from build123d import *

# Parameters (mm, degrees)
EXTRUIR1_DEPTH            = 5.5
EXTRUIR2_DEPTH            = 2
EXTRUIR3_DEPTH            = 2
CROQUIS5_R                = 1
EXTRUIR4_DEPTH            = 41.608650556
VACIADO1_DEPTH            = 2
VACIADO1_START            = 2
VACIADO1_2_DEPTH          = 2
CROQUIS8_W                = 4
CROQUIS8_H                = 1
EXTRUIR7_DEPTH            = 3
SIMETR_A3_COPY_1_SKETCH_W = 4
SIMETR_A3_COPY_1_SKETCH_H = 1
SIMETR_A3_COPY_1_DEPTH    = 3
REDONDEO1_R               = 0.5
CROQUIS9_W                = 5
CROQUIS9_H                = 7.4
EXTRUIR8_DEPTH            = 41.707032562


# Read off the part's stored shape, not the designer's step: Vaciado1
with BuildPart() as part:
    # Croquis2 → Extruir1 (new body)
    with BuildSketch(Plane(origin=(0, 0, 0), x_dir=(0, 0, -1), z_dir=(1, 0, 0))):
        with BuildLine():
            Line((-37, 8.75), (37, 8.75))
            ThreePointArc((37, 8.75), (38.767766953, 8.017766953), (39.5, 6.25))
            Line((39.5, 6.25), (39.5, -6.25))
            ThreePointArc((39.5, -6.25), (38.767766953, -8.017766953), (37, -8.75))
            Line((37, -8.75), (-37, -8.75))
            ThreePointArc((-37, -8.75), (-38.767766953, -8.017766953), (-39.5, -6.25))
            Line((-39.5, -6.25), (-39.5, 6.25))
            ThreePointArc((-39.5, 6.25), (-38.767766953, 8.017766953), (-37, 8.75))
        make_face()
    extrude(amount=EXTRUIR1_DEPTH)

    # Croquis3 → Extruir2 (cut)
    with BuildSketch(Plane(origin=(5.5, 0, 0), x_dir=(0, 0, -1), z_dir=(1, 0, 0))):
        with BuildLine():
            Line((-32, 6.75), (32, 6.75))
            ThreePointArc((32, 6.75), (33.060660172, 6.310660172), (33.5, 5.25))
            Line((33.5, 5.25), (33.5, -5.25))
            ThreePointArc((33.5, -5.25), (33.060660172, -6.310660172), (32, -6.75))
            Line((32, -6.75), (-32, -6.75))
            ThreePointArc((-32, -6.75), (-33.060660172, -6.310660172), (-33.5, -5.25))
            Line((-33.5, -5.25), (-33.5, 5.25))
            ThreePointArc((-33.5, 5.25), (-33.060660172, 6.310660172), (-32, 6.75))
        make_face()
    extrude(amount=-EXTRUIR2_DEPTH, mode=Mode.SUBTRACT)

    # Croquis4 → Extruir3 (cut)
    with BuildSketch(Plane(origin=(5.5, 0, 0), x_dir=(0, 0, -1), z_dir=(1, 0, 0))):
        with BuildLine():
            Line((-39.5, 2.5), (-37.32, 2.5))
            ThreePointArc((-37.32, 2.5), (-34.82, 0), (-37.32, -2.5))
            Line((-37.32, -2.5), (-39.5, -2.5))
            Line((-39.5, -2.5), (-39.5, 2.5))
        make_face()
    extruir3 = extrude(amount=-EXTRUIR3_DEPTH, mode=Mode.SUBTRACT)

    # Croquis5 → Extruir4 (cut, through all)
    with BuildSketch(Plane(origin=(3.5, 0, 0), x_dir=(0, 0, -1), z_dir=(1, 0, 0))):
        with Locations((-37.32, 0)):
            Circle(CROQUIS5_R)
    extruir4 = extrude(amount=-EXTRUIR4_DEPTH, mode=Mode.SUBTRACT)

    # Simetría1: Extruir3, Extruir4 across plane
    add(extruir3.mirror(Plane.XY), mode=Mode.SUBTRACT)
    add(extruir4.mirror(Plane.XY), mode=Mode.SUBTRACT)

    # Vaciado1 outline → Vaciado1 (cut)
    with BuildSketch(Plane.YZ):
        with BuildLine():
            ThreePointArc((-7.25, -37), (-6.957106781, -37.707106781), (-6.25, -38))
            Line((-6.25, -38), (-2.405743128, -38))
            ThreePointArc((-2.405743128, -38), (0, -34.82), (2.405743128, -38))
            Line((2.405743128, -38), (6.25, -38))
            ThreePointArc((6.25, -38), (6.957106781, -37.707106781), (7.25, -37))
            Line((7.25, -37), (7.25, 37))
            ThreePointArc((7.25, 37), (6.957106781, 37.707106781), (6.25, 38))
            Line((6.25, 38), (2.405743128, 38))
            ThreePointArc((2.405743128, 38), (0, 34.82), (-2.405743128, 38))
            Line((-2.405743128, 38), (-6.25, 38))
            ThreePointArc((-6.25, 38), (-6.957106781, 37.707106781), (-7.25, 37))
            Line((-7.25, 37), (-7.25, -37))
        make_face()
    extrude(amount=VACIADO1_DEPTH, mode=Mode.SUBTRACT)

    # Vaciado1 2 outline → Vaciado1 2 (cut)
    with BuildSketch(Plane.YZ.offset(VACIADO1_START)):
        with BuildLine():
            Line((-7.25, -34.236067977), (-7.25, -37))
            ThreePointArc((-7.25, -37), (-6.957106781, -37.707106781), (-6.25, -38))
            Line((-6.25, -38), (-4, -38))
            Line((-4, -38), (-4, -37.32))
            ThreePointArc((-4, -37.32), (-3.810109158, -36.102187122), (-3.258465897, -35))
            Line((-3.258465897, -35), (-5.25, -35))
            ThreePointArc((-5.25, -35), (-6.320466269, -34.802517077), (-7.25, -34.236067977))
        make_face()
        with BuildLine():
            Line((-7.25, 37), (-7.25, 34.236067977))
            ThreePointArc((-7.25, 34.236067977), (-6.320466269, 34.802517077), (-5.25, 35))
            Line((-5.25, 35), (-3.258465897, 35))
            ThreePointArc((-3.258465897, 35), (-3.810109158, 36.102187122), (-4, 37.32))
            Line((-4, 37.32), (-4, 38))
            Line((-4, 38), (-6.25, 38))
            ThreePointArc((-6.25, 38), (-6.957106781, 37.707106781), (-7.25, 37))
        make_face()
        with BuildLine():
            Line((4, -37.32), (4, -38))
            Line((4, -38), (6.25, -38))
            ThreePointArc((6.25, -38), (6.957106781, -37.707106781), (7.25, -37))
            Line((7.25, -37), (7.25, -34.236067977))
            ThreePointArc((7.25, -34.236067977), (6.320466269, -34.802517077), (5.25, -35))
            Line((5.25, -35), (3.258465897, -35))
            ThreePointArc((3.258465897, -35), (3.810109158, -36.102187122), (4, -37.32))
        make_face()
        with BuildLine():
            Line((6.25, 38), (4, 38))
            Line((4, 38), (4, 37.32))
            ThreePointArc((4, 37.32), (3.810109158, 36.102187122), (3.258465897, 35))
            Line((3.258465897, 35), (5.25, 35))
            ThreePointArc((5.25, 35), (6.320466269, 34.802517077), (7.25, 34.236067977))
            Line((7.25, 34.236067977), (7.25, 37))
            ThreePointArc((7.25, 37), (6.957106781, 37.707106781), (6.25, 38))
        make_face()
    extrude(amount=VACIADO1_2_DEPTH, mode=Mode.SUBTRACT)

    # Croquis8 → Extruir7 (add)
    with BuildSketch(Plane.ZY.offset(-2)):
        with Locations((-20.5, 7.65)):
            Rectangle(CROQUIS8_W, CROQUIS8_H)
    extruir7 = extrude(amount=EXTRUIR7_DEPTH)

    # Simetría2: Extruir7 across plane
    add(extruir7.mirror(Plane.XY))

    # Simetría3: Extruir7 across plane
    add(extruir7.mirror(Plane.ZX))

    # Simetría3 copy 1 sketch → Simetría3 copy 1 (add)
    with BuildSketch(Plane(origin=(2, 0, 0), x_dir=(0, 0, -1), z_dir=(-1, 0, 0))):
        with Locations((-20.5, 7.65)):
            Rectangle(SIMETR_A3_COPY_1_SKETCH_W, SIMETR_A3_COPY_1_SKETCH_H)
    extrude(amount=SIMETR_A3_COPY_1_DEPTH)

    # Redondeo1
    redondeo1_edges = [part.edges().sort_by_distance(p)[0] for p in [
        (5.5, -8.017766953, 38.767766953),
        (5.5, -8.75, 0),
        (5.5, -8.017766953, -38.767766953),
        (5.5, -4.375, -39.5),
        (5.5, 8.017766953, -38.767766953),
        (5.5, 8.75, 0),
        (5.5, 8.017766953, 38.767766953),
        (5.5, -4.375, 39.5),
        (5.5, -2.5, 38.41),
        (5.5, 0, 34.82),
        (5.5, 2.5, 38.41),
        (5.5, 4.375, 39.5),
        (5.5, 4.375, -39.5),
        (5.5, -2.5, -38.41),
        (5.5, 0, -34.82),
        (5.5, 2.5, -38.41),
    ]]
    fillet(redondeo1_edges, radius=REDONDEO1_R)

    # Croquis9 → Extruir8 (cut, through all)
    with BuildSketch(Plane(origin=(3.5, 0, 0), x_dir=(0, 0, -1), z_dir=(1, 0, 0))):
        with Locations((-23.987, 1.8)):
            Rectangle(CROQUIS9_W, CROQUIS9_H)
        with BuildLine():
            Line((-4.0245, 0.401469998), (-4.0245, 1.2))
            ThreePointArc((-4.0245, 1.2), (-3.819474747, 1.694974747), (-3.3245, 1.9))
            Line((-3.3245, 1.9), (2.9755, 1.9))
            ThreePointArc((2.9755, 1.9), (3.470474747, 1.694974747), (3.6755, 1.2))
            Line((3.6755, 1.2), (3.6755, 0.401469998))
            ThreePointArc((3.6755, 0.401469998), (3.622215673, 0.133591595), (3.470474747, -0.093504749))
            Line((3.470474747, -0.093504749), (3.246579496, -0.3174))
            ThreePointArc((3.246579496, -0.3174), (3.18154767, -0.414727005), (3.15871153, -0.529532034))
            Line((3.15871153, -0.529532034), (3.15871153, -1.3))
            ThreePointArc((3.15871153, -1.3), (2.953686277, -1.794974747), (2.45871153, -2))
            Line((2.45871153, -2), (-2.80771153, -2))
            ThreePointArc((-2.80771153, -2), (-3.302686277, -1.794974747), (-3.50771153, -1.3))
            Line((-3.50771153, -1.3), (-3.50771153, -0.529532034))
            ThreePointArc((-3.50771153, -0.529532034), (-3.53054767, -0.414727005), (-3.595579496, -0.3174))
            Line((-3.595579496, -0.3174), (-3.819474747, -0.093504749))
            ThreePointArc((-3.819474747, -0.093504749), (-3.971215673, 0.133591595), (-4.0245, 0.401469998))
        make_face()
    extrude(amount=-EXTRUIR8_DEPTH, mode=Mode.SUBTRACT)


solid = part.part
Build history of the part. All positions in model axes, mm. A direction names the side the tool comes from. Coordinates: 2 decimals unless noted, no trailing zeros. Order: outer loops, then holes, each group sorted by start corner. A loop starts at its lowest first (then second) coordinate and runs counter-clockwise, first axis right, second up. Notation, with made-up numbers: (21.25, 59.25) - (48.25, 59.25) arc R35 cw to (48.25, 97.25) - close; hole circle Ø2 at (77.5, 56.25). An arc over 180 degrees is marked (long way). Write item = value, one per line. Start each with the question number.
1) Wall check: line 1 along Y through (x, z) = (1.5, 17); line 2 along Z through (x, y) = (4.5, 3.5); line 3 along X through (y, z) = (3.75, -3.5). Give the ranges that are in metal, low to high. Write a range as from..to.
2) Saw through at B-B on x = 0.75. Count the separate pieces of the cut face and the enclosed holes in it, then the cut area to 3 significant figures.
3) Saw through at A-A on z = -26. Write the cut outline in (x, y).
4) Two-plate mould, pull along Z, no slides. Class faces 4 (the face through (5, -6.75, 0)), 5 (the face through (2.465, -8.037, 38.748)), 6 (the face through (3, -4, -35)), 7 (the face through (2, 8.75, 1)): pulls with the +Z half, pulls with the -Z half, needs draft (parallel to the pull), parting line crosses it, or undercut.
5) Flat gauge pins, fed straight in: pin 1 Ø0.6 at (x, y) = (5, 0.5) entering from +Z; pin 2 Ø0.6 at (x, y) = (4.5, 1.5) entering from -Z; pin 3 Ø1.5 at (y, z) = (-5, 5) entering from -X. Where does each tip first touch, or does it go through?
6) 3-axis set-ups, long thin cutter, end or side, ignore diameter. For faces 1 (the face through (3, 5.5, 24)), 2 (the face through (1, 7.25, 0)), 3 (the face through (4, 2.5, 38)): which of +Z, -Z, +X, -X, +Y, -Y reach the whole face in a straight line?
From the geometry:
q1.line_1 = -8.75..-7.25, 7.25..8.75
q1.line_2 = -39.5..-33.5, 33.5..39.5
q1.line_3 = 2..3.5
q2.separate_pieces = 1
q2.enclosed_holes = 3
q2.area = 298 mm^2
q3.outline = (0, -8.75) - (5, -8.75) arc R0.5 ccw to (5.5, -8.25) - (5.5, -6.75) - (3.5, -6.75) - (3.5, 6.75) - (5.5, 6.75) - (5.5, 8.25) arc R0.5 ccw to (5, 8.75) - (0, 8.75) - (0, 7.25) - (2, 7.25) - (2, -7.25) - (0, -7.25) - close
q4.face_4 = undercut
q4.face_5 = pulls with the +Z half
q4.face_6 = undercut
q4.face_7 = needs draft
q5.pin_1 = 34.95
q5.pin_2 = -35.59
q5.pin_3 = 2
q6.face_1 = +X, -X
q6.face_2 = -X
q6.face_3 = +Z, +X
